Read the model definition and answer for the solid it produces. Units are mm, in the model's axes. A direction names the side the tool comes from. Round coordinates to 2 decimals unless told otherwise and drop trailing zeros. Order: outer loops, then holes, each group sorted by start corner. A loop starts at its lowest first (then second) coordinate and runs counter-clockwise, first axis right, second up.
from build123d import *

# Parameters (mm, degrees)
BOSS_EXTRUDE1_DEPTH                             = 14
SKETCH3_R                                       = 4.125
CUT_EXTRUDE1_DEPTH                              = 8.8
SKETCH8_R                                       = 2.7
CUT_EXTRUDE3_DEPTH                              = 49.958231273
SKETCH11_W                                      = 49
SKETCH11_H                                      = 0.5
CUT_EXTRUDE6_DEPTH                              = 49.958231273
BOSS_EXTRUDE2_START                             = -4
SKETCH12_R                                      = 2.7
SKETCH12_R_2                                    = 1.5
SKETCH12_R_3                                    = 1.8
BOSS_EXTRUDE2_DEPTH                             = 4
CUT_EXTRUDE7_DEPTH                              = 2
BOSS_EXTRUDE3_START                             = 5
SKETCH18_R                                      = 2.7
SKETCH18_R_2                                    = 2.4
BOSS_EXTRUDE3_DEPTH                             = 5
SKETCH17_R                                      = 2.3
SKETCH17_W                                      = 11.431818182
SKETCH17_H                                      = 0.1
CUT_EXTRUDE8_DEPTH                              = 22
BOSS_EXTRUDE4_DEPTH                             = 4
BOSS_EXTRUDE4_DEPTH_BACK                        = 10
SKETCH20_W                                      = 9.5
SKETCH20_H                                      = 11
SKETCH20_R                                      = 2.7
SKETCH20_R_2                                    = 2.55
CUT_EXTRUDE9_START                              = -10
SKETCH21_R                                      = 2.55
SKETCH21_R_2                                    = 2.7
CUT_EXTRUDE9_DEPTH                              = 10
CSK_FOR_M3_FLAT_HEAD_MACHINE_SCREW1_D           = 3.4
CSK_FOR_M3_FLAT_HEAD_MACHINE_SCREW1_CSINK_D     = 6.3
CSK_FOR_M3_FLAT_HEAD_MACHINE_SCREW1_CSINK_ANGLE = 90


with BuildPart() as part:
    # Sketch2 → Boss-Extrude1 (new body)
    with BuildSketch(Plane.XY):
        Polygon((12.982187117, 18.175494031), (23.982187117, 18.175494031), (42.982187117, 26.975494031), (42.982187117, 36.975494031), (-6.017812883, 36.975494031), (-6.017812883, 26.975494031), align=None)
    extrude(amount=BOSS_EXTRUDE1_DEPTH)

    # Sketch3 → Cut-Extrude1 (cut)
    with BuildSketch(Plane.XZ.offset(-18.175494031)):
        with Locations(Location((18.482187117, 7, 0), (0, 0, 270))):
            Circle(SKETCH3_R)
    extrude(amount=-CUT_EXTRUDE1_DEPTH, mode=Mode.SUBTRACT)

    # Sketch8 → Cut-Extrude3 (cut, through all)
    with BuildSketch(Plane.XZ.offset(-18.175494031)):
        with Locations(Location((37.482187117, 7, 0), (0, 0, 270))):
            Circle(SKETCH8_R)
        with Locations(Location((-0.517812883, 7, 0), (0, 0, 270))):
            Circle(SKETCH8_R)
    extrude(amount=-CUT_EXTRUDE3_DEPTH, mode=Mode.SUBTRACT)

    # Sketch11 → Cut-Extrude6 (cut, through all)
    with BuildSketch(Plane.XZ.offset(-18.175494031)):
        with Locations((18.482187117, 13.75)):
            Rectangle(SKETCH11_W, SKETCH11_H)
        with Locations((18.482187117, 0.25)):
            Rectangle(SKETCH11_W, SKETCH11_H)
    extrude(amount=-CUT_EXTRUDE6_DEPTH, mode=Mode.SUBTRACT)

    # Sketch12 → Boss-Extrude2 (add)
    # profile 1 of 2: a face of its own
    with BuildSketch(Plane(origin=(0, 36.975494031, 0), x_dir=(1, 0, 0), z_dir=(0, 1, 0)).offset(BOSS_EXTRUDE2_START)):
        with Locations((-0.517812883, -7)):
            Circle(SKETCH12_R)
        with Locations(Location((-0.517812883, -7, 0), (0, 0, 270))):
            Circle(SKETCH12_R_2, mode=Mode.SUBTRACT)
    # profile 2 of 2: a face of its own
    with BuildSketch(Plane(origin=(0, 36.975494031, 0), x_dir=(1, 0, 0), z_dir=(0, 1, 0)).offset(BOSS_EXTRUDE2_START)):
        with Locations(Location((37.482187117, -7, 0), (0, 0, 180))):
            Circle(SKETCH12_R)
        with Locations(Location((37.482187117, -7, 0), (0, 0, 270))):
            Circle(SKETCH12_R_3, mode=Mode.SUBTRACT)
    extrude(amount=BOSS_EXTRUDE2_DEPTH)

    # Sketch15 → Cut-Extrude7 (cut)
    with BuildSketch(Plane(origin=(0, 0, 0.5), x_dir=(-1, 0, 0), z_dir=(0, 0, -1))):
        Polygon((-33.482187117, 22.575494031), (-33.482187117, 36.975494031), (-3.482187117, 36.975494031), (-3.482187117, 22.575494031), (-12.982187117, 18.175494031), (-23.982187117, 18.175494031), align=None)
    extrude(amount=-CUT_EXTRUDE7_DEPTH, mode=Mode.SUBTRACT)

    # Sketch18 → Boss-Extrude3 (add)
    # profile 1 of 2: a face of its own
    with BuildSketch(Plane.XZ.offset(-32.975494031).offset(BOSS_EXTRUDE3_START)):
        with Locations(Location((37.482187117, 7, 0), (0, 0, 270))):
            Circle(SKETCH18_R)
        with Locations(Location((37.482187117, 7, 0), (0, 0, 270))):
            Circle(SKETCH18_R_2, mode=Mode.SUBTRACT)
    # profile 2 of 2: a face of its own
    with BuildSketch(Plane.XZ.offset(-32.975494031).offset(BOSS_EXTRUDE3_START)):
        with Locations(Location((-0.517812883, 7, 0), (0, 0, 270))):
            Circle(SKETCH18_R)
        with Locations(Location((-0.517812883, 7, 0), (0, 0, 270))):
            Circle(SKETCH18_R_2, mode=Mode.SUBTRACT)
    extrude(amount=-BOSS_EXTRUDE3_DEPTH)

    # Sketch17 → Cut-Extrude8 (cut)
    with BuildSketch(Plane(origin=(0, 0, 2.5), x_dir=(-1, 0, 0), z_dir=(0, 0, -1))):
        with Locations((-18.482187117, 31.475494031)):
            Circle(SKETCH17_R)
        with Locations((-18.482187117, 18.225494031)):
            Rectangle(SKETCH17_W, SKETCH17_H)
    extrude(amount=-CUT_EXTRUDE8_DEPTH, mode=Mode.SUBTRACT)

    # Sketch20 → Boss-Extrude4 (add, two sides: drawn at the far end of the back side and taken through both)
    # profile 1 of 2: a face of its own
    with BuildSketch(Plane(origin=(0, 26.975494031, 0), x_dir=(-1, 0, 0), z_dir=(0, -1, 0)).offset(-BOSS_EXTRUDE4_DEPTH_BACK)):
        with Locations((-38.232187117, -8)):
            Rectangle(SKETCH20_W, SKETCH20_H)
        with Locations(Location((-37.482187117, -7, 0), (0, 0, 90))):
            Circle(SKETCH20_R, mode=Mode.SUBTRACT)
    # profile 2 of 2: a face of its own
    with BuildSketch(Plane(origin=(0, 26.975494031, 0), x_dir=(-1, 0, 0), z_dir=(0, -1, 0)).offset(-BOSS_EXTRUDE4_DEPTH_BACK)):
        with Locations((1.267812883, -8)):
            Rectangle(SKETCH20_W, SKETCH20_H)
        with Locations(Location((0.517812883, -7, 0), (0, 0, 90))):
            Circle(SKETCH20_R_2, mode=Mode.SUBTRACT)
    extrude(amount=BOSS_EXTRUDE4_DEPTH + BOSS_EXTRUDE4_DEPTH_BACK)

    # Sketch21 → Cut-Extrude9 (cut)
    with BuildSketch(Plane.XZ.offset(-22.975494031).offset(CUT_EXTRUDE9_START)):
        with Locations(Location((-0.517812883, 7, 0), (0, 0, 270))):
            Circle(SKETCH21_R)
        with Locations(Location((37.482187117, 7, 0), (0, 0, 270))):
            Circle(SKETCH21_R_2)
    extrude(amount=CUT_EXTRUDE9_DEPTH, mode=Mode.SUBTRACT)

    # CSK for M3 Flat Head Machine Screw1 (through all)
    with Locations(Plane(origin=(0, 36.975494031, 0), x_dir=(1, 0, 0), z_dir=(0, 1, 0))):
        with Locations((-0.517812883, -7), (37.482187117, -7)):
            CounterSinkHole(CSK_FOR_M3_FLAT_HEAD_MACHINE_SCREW1_D / 2, CSK_FOR_M3_FLAT_HEAD_MACHINE_SCREW1_CSINK_D / 2, counter_sink_angle=CSK_FOR_M3_FLAT_HEAD_MACHINE_SCREW1_CSINK_ANGLE)


solid = part.part
Q1. Straight lines are drawn through the part: probe 1 along X at (y, z) = (34.35, 7); probe 2 along X at (y, z) = (23.5, 7); probe 3 along Z at (x, y) = (18.5, 23.5). For each, find the intervals that lie inside material, in ascending order.
Outcome:
probe 1: x = -6.02 to -2.22, 1.18 to 35.68, 39.28 to 42.98
probe 2: x = -6.02 to -3.07, 2.03 to 14.36, 22.61 to 34.78, 40.18 to 42.98
probe 3: z = 2.5 to 2.88, 11.12 to 13.5
Q2. Flat-ended cylindrical pins translate along their axes: pin 1 (6 mm diameter, centred on x = 37.48, z = 7, fed in from -Y); pin 2 (7 mm diameter, centred on x = 37.5, z = 9, fed in from -Y); pin 3 (2 mm diameter, centred on x = -0.52, z = 7, fed in from -Y); pin 4 (3 mm diameter, centred on x = 11, z = 8.5, fed in from -Y). Find the tip coordinate at first contact, or state that the pin passes through.
Outcome:
pin 1: stops at y = 22.98
pin 2: stops at y = 22.82
pin 3: passes through
pin 4: stops at y = 18.4
Q3. For a pull along Z with two mould halves and no side action, classify faces 1 (the face through (20.31, 30.08, 7.92)), 2 (the face through (-0.15, 34.23, 8.66)), 3 (the face through (-1, 31, 0.5)) as released by +Z, released by -Z, zero draft, split by the parting line, or undercut.
Outcome:
face 1: zero draft
face 2: undercut
face 3: released by -Z
Q4. A cutting plane is placed at B-B, the plane z = 7. Give the number of separate pieces and of enclosed holes in the cut face, plus the area to 3 significant figures.
Outcome:
separate pieces: 3
enclosed holes: 1
area: 562 mm2
Q5. A cutting plane is placed at C-C, the plane y = 21.25. Give the vertices of the cut face in (x, z) (3 decimals).
Outcome:
outline: (6.344, 2.5) - (30.62, 2.5) - (30.62, 13.5) - (6.344, 13.5) - close; hole circle Ø8.25 at (18.482, 7)
Q6. A cutting plane is placed at A-A, the plane y = 32.25. Give the vertices of the cut face in (x, z), plus the area to 3 significant figures.
Outcome:
outline: (-6.02, 0.5) - (3.48, 0.5) - (3.48, 2.5) - (16.32, 2.5) - (16.32, 13.5) - (-6.02, 13.5) - close; (20.65, 2.5) - (33.48, 2.5) - (33.48, 0.5) - (42.98, 0.5) - (42.98, 13.5) - (20.65, 13.5) - close; hole circle Ø5.1 at (-0.52, 7); hole circle Ø5.4 at (37.48, 7)
area: 486 mm2
Q7. For faces 4 (the face through (3.482, 30, 1)), 5 (the face through (-3, 22.975, 9)), 6 (the face through (-4, 24, 2.5)), 7 (the face through (40, 22.975, 9)), 8 (the face through (41, 24, 2.5)), determine the directions among +Z, -Z, +X, -X, +Y, -Y from which every point of the face is accessible in a straight line to the end or side of a thin tool.
Outcome:
face 4: -Z, +Y, -Y
face 5: +Z, -Z, -X, -Y
face 6: -Z, -X, -Y
face 7: +Z, -Z, +X, -Y
face 8: -Z, +X, -Y
Q8. A cutting plane is placed at D-D, the plane x = 26.5. Give the vertices of the cut face in (y, z).
Outcome:
outline: (19.34, 2.5) - (36.98, 2.5) - (36.98, 13.5) - (19.34, 13.5) - close
